Here's how the part is built. I have some questions about the finished solid (model axes, mm). A direction names the side the tool comes from. Give positions to 0.01 mm unless a question says otherwise; leave off trailing zeros. Write each loop counter-clockwise with the first axis right and the second up, starting at its lowest first coordinate (ties: lowest second). Pieces come first, ordered by that corner, then holes. Notation, with made-up numbers: (21, -35) -> (62, -35) arc R14 ccw to (62, -8) -> close; hole circle Ø6 at (-37, 38.5). An arc over 180 degrees is marked (long way). Use one line per item in the form item = value.
```python
from build123d import *

# Parameters (mm, degrees)
BOSS_EXTRUDE1_DEPTH = 56.75
SKETCH2_W           = 5
SKETCH2_H           = 85
SKETCH2_R           = 1.5
CUT_EXTRUDE1_DEPTH  = 2
SKETCH3_R           = 5
CUT_EXTRUDE2_DEPTH  = 3
CHAMFER1_SIZE       = 0.5
CUT_EXTRUDE3_DEPTH  = 5.5
CUT_EXTRUDE4_DEPTH  = 10


with BuildPart() as part:
    # Sketch1 → Boss-Extrude1 (new body, symmetric)
    with BuildSketch(Plane.XY):
        Polygon((0, 50), (0, -50), (7.5, -50), (7.5, -42.5), (2, -42.5), (2, 42.5), (7.5, 42.5), (7.5, 50), align=None)
    extrude(amount=BOSS_EXTRUDE1_DEPTH, both=True)

    # Sketch2 → Cut-Extrude1 (cut)
    with BuildSketch(Plane(origin=(2, 0, 0), x_dir=(0, 0, -1), z_dir=(1, 0, 0))):
        with Locations((-54.25, 0)):
            Rectangle(SKETCH2_W, SKETCH2_H)
        with Locations((54.25, 0)):
            Rectangle(SKETCH2_W, SKETCH2_H)
        with Locations((-47.75, 17.5)):
            Circle(SKETCH2_R)
        with Locations((-47.75, -17.5)):
            Circle(SKETCH2_R)
        with Locations((47.75, 17.5)):
            Circle(SKETCH2_R)
        with Locations((47.75, -17.5)):
            Circle(SKETCH2_R)
    extrude(amount=-CUT_EXTRUDE1_DEPTH, mode=Mode.SUBTRACT)

    # Sketch3 → Cut-Extrude2 (cut, through all)
    with BuildSketch(Plane(origin=(2, 0, 0), x_dir=(0, 0, -1), z_dir=(1, 0, 0))):
        Circle(SKETCH3_R)
        with BuildLine():
            Line((-30.354626116, -39.5), (25.154965406, -39.5))
            ThreePointArc((25.154965406, -39.5), (29.821654194, -36.294997423), (28.505643146, -30.7888063))
            Line((28.505643146, -30.7888063), (7.843483172, -12.13382758))
            ThreePointArc((7.843483172, -12.13382758), (6.353277021, -11.405989443), (4.704093974, -11.58108371))
            ThreePointArc((4.704093974, -11.58108371), (0, -12.5), (-4.704093974, -11.58108371))
            ThreePointArc((-4.704093974, -11.58108371), (-6.353277021, -11.405989443), (-7.843483172, -12.13382758))
            Line((-7.843483172, -12.13382758), (-32.36503276, -34.27328378))
            ThreePointArc((-32.36503276, -34.27328378), (-33.154639389, -37.576998454), (-30.354626116, -39.5))
        make_face()
        with BuildLine():
            Line((-43.75, -27.697319579), (-43.75, 27.697319579))
            ThreePointArc((-43.75, 27.697319579), (-41.968355463, 30.438780862), (-38.739593356, 29.924035799))
            Line((-38.739593356, 29.924035799), (-12.869499782, 6.56703703))
            ThreePointArc((-12.869499782, 6.56703703), (-11.993687913, 5.158698897), (-11.999924538, 3.500258718))
            ThreePointArc((-11.999924538, 3.500258718), (-12.5, 0), (-11.999924538, -3.500258718))
            ThreePointArc((-11.999924538, -3.500258718), (-11.993687913, -5.158698897), (-12.869499782, -6.56703703))
            Line((-12.869499782, -6.56703703), (-38.739593356, -29.924035799))
            ThreePointArc((-38.739593356, -29.924035799), (-41.968355463, -30.438780862), (-43.75, -27.697319579))
        make_face()
        with BuildLine():
            Line((-30.354626116, 39.5), (25.154965406, 39.5))
            ThreePointArc((25.154965406, 39.5), (29.821654194, 36.294997423), (28.505643146, 30.7888063))
            Line((28.505643146, 30.7888063), (7.843483172, 12.13382758))
            ThreePointArc((7.843483172, 12.13382758), (6.353277021, 11.405989443), (4.704093974, 11.58108371))
            ThreePointArc((4.704093974, 11.58108371), (0, 12.5), (-4.704093974, 11.58108371))
            ThreePointArc((-4.704093974, 11.58108371), (-6.353277021, 11.405989443), (-7.843483172, 12.13382758))
            Line((-7.843483172, 12.13382758), (-32.36503276, 34.27328378))
            ThreePointArc((-32.36503276, 34.27328378), (-33.154639389, 37.576998454), (-30.354626116, 39.5))
        make_face()
        with BuildLine():
            Line((43.75, -27.697319579), (43.75, 27.697319579))
            ThreePointArc((43.75, 27.697319579), (41.968355463, 30.438780862), (38.739593356, 29.924035799))
            Line((38.739593356, 29.924035799), (12.869499782, 6.56703703))
            ThreePointArc((12.869499782, 6.56703703), (11.993687913, 5.158698897), (11.999924538, 3.500258718))
            ThreePointArc((11.999924538, 3.500258718), (12.5, 0), (11.999924538, -3.500258718))
            ThreePointArc((11.999924538, -3.500258718), (11.993687913, -5.158698897), (12.869499782, -6.56703703))
            Line((12.869499782, -6.56703703), (38.739593356, -29.924035799))
            ThreePointArc((38.739593356, -29.924035799), (41.968355463, -30.438780862), (43.75, -27.697319579))
        make_face()
        with BuildLine():
            Line((35.25, -39.45), (38.25, -39.45))
            ThreePointArc((38.25, -39.45), (39.8, -41), (38.25, -42.55))
            Line((38.25, -42.55), (35.25, -42.55))
            ThreePointArc((35.25, -42.55), (33.7, -41), (35.25, -39.45))
        make_face()
        with BuildLine():
            Line((35.25, 42.55), (38.25, 42.55))
            ThreePointArc((38.25, 42.55), (39.8, 41), (38.25, 39.45))
            Line((38.25, 39.45), (35.25, 39.45))
            ThreePointArc((35.25, 39.45), (33.7, 41), (35.25, 42.55))
        make_face()
    extrude(amount=-CUT_EXTRUDE2_DEPTH, mode=Mode.SUBTRACT)

    # Chamfer1
    chamfer1_edges = [part.edges().sort_by_distance(p)[0] for p in [
        (0, -50, 0),
        (0, 50, 0),
    ]]
    chamfer(chamfer1_edges, length=CHAMFER1_SIZE)

    # Sketch4 → Cut-Extrude3 (cut)
    with BuildSketch(Plane(origin=(7.5, 0, 0), x_dir=(0, 0, -1), z_dir=(1, 0, 0))):
        with BuildLine():
            Line((42.75, -48), (-42.75, -48))
            ThreePointArc((-42.75, -48), (-45.578427125, -46.828427125), (-46.75, -44))
            Line((-46.75, -44), (-46.75, -43.5))
            ThreePointArc((-46.75, -43.5), (-47.042893219, -42.792893219), (-47.75, -42.5))
            Line((-47.75, -42.5), (47.75, -42.5))
            ThreePointArc((47.75, -42.5), (47.042893219, -42.792893219), (46.75, -43.5))
            Line((46.75, -43.5), (46.75, -44))
            ThreePointArc((46.75, -44), (45.578427125, -46.828427125), (42.75, -48))
        make_face()
        with BuildLine():
            Line((-46.75, 44), (-46.75, 43.5))
            ThreePointArc((-46.75, 43.5), (-47.042893219, 42.792893219), (-47.75, 42.5))
            Line((-47.75, 42.5), (47.75, 42.5))
            ThreePointArc((47.75, 42.5), (47.042893219, 42.792893219), (46.75, 43.5))
            Line((46.75, 43.5), (46.75, 44))
            ThreePointArc((46.75, 44), (45.578427125, 46.828427125), (42.75, 48))
            Line((42.75, 48), (-42.75, 48))
            ThreePointArc((-42.75, 48), (-45.578427125, 46.828427125), (-46.75, 44))
        make_face()
    extrude(amount=-CUT_EXTRUDE3_DEPTH, mode=Mode.SUBTRACT)

    # Sketch5 → Cut-Extrude4 (cut)
    with BuildSketch(Plane.ZY):
        with BuildLine():
            ThreePointArc((-51.75, 27.820508076), (-51.409258263, 30.408698527), (-50.410254038, 32.820508076))
            Line((-50.410254038, 32.820508076), (-48.285898385, 36.5))
            ThreePointArc((-48.285898385, 36.5), (-48.285898385, 40.5), (-51.75, 42.5))
            Line((-51.75, 42.5), (-51.75, 27.820508076))
        make_face()
        with BuildLine():
            ThreePointArc((-50.410254038, -32.820508076), (-51.409258263, -30.408698527), (-51.75, -27.820508076))
            Line((-51.75, -27.820508076), (-51.75, -42.5))
            ThreePointArc((-51.75, -42.5), (-48.285898385, -40.5), (-48.285898385, -36.5))
            Line((-48.285898385, -36.5), (-50.410254038, -32.820508076))
        make_face()
    cut_extrude4 = extrude(amount=-CUT_EXTRUDE4_DEPTH, mode=Mode.SUBTRACT)

    # Mirror1: Cut-Extrude4 across plane
    add(cut_extrude4.mirror(Plane.XY), mode=Mode.SUBTRACT)


solid = part.part
```
Q1. I want a section at C-C, the plane z = 28. Write out the boundary of the cut face in (x, y).
Result set:
outline = (0, -49.5) -> (0.5, -50) -> (7.5, -50) -> (7.5, -48) -> (2, -48) -> (2, -39.5) -> (0, -39.5) -> close; (0, -30.33) -> (2, -30.33) -> (2, -20.23) -> (0, -20.23) -> close; (0, 20.23) -> (2, 20.23) -> (2, 30.33) -> (0, 30.33) -> close; (0, 39.5) -> (2, 39.5) -> (2, 48) -> (7.5, 48) -> (7.5, 50) -> (0.5, 50) -> (0, 49.5) -> close
Q2. I want a section at A-A, the plane x = 3.75. Write out the boundary of the cut face in (y, z).
Result set:
outline = (-50, -56.75) -> (-42.5, -56.75) -> (-42.5, -47.75) arc R1 ccw to (-43.5, -46.75) -> (-44, -46.75) arc R4 cw to (-48, -42.75) -> (-48, 42.75) arc R4 cw to (-44, 46.75) -> (-43.5, 46.75) arc R1 ccw to (-42.5, 47.75) -> (-42.5, 56.75) -> (-50, 56.75) -> close; (42.5, -56.75) -> (50, -56.75) -> (50, 56.75) -> (42.5, 56.75) -> (42.5, 47.75) arc R1 ccw to (43.5, 46.75) -> (44, 46.75) arc R4 cw to (48, 42.75) -> (48, -42.75) arc R4 cw to (44, -46.75) -> (43.5, -46.75) arc R1 ccw to (42.5, -47.75) -> close
Q3. I want a section at B-B, the plane y = -25.5. Write out the boundary of the cut face in (x, z).
Result set:
outline = (0, -51.75) -> (2, -51.75) -> (2, -43.75) -> (0, -43.75) -> close; (0, -33.84) -> (2, -33.84) -> (2, -22.65) -> (0, -22.65) -> close; (0, 22.65) -> (2, 22.65) -> (2, 33.84) -> (0, 33.84) -> close; (0, 43.75) -> (2, 43.75) -> (2, 51.75) -> (0, 51.75) -> close
Q4. Will these pins go through, and if not, where does the flat tip stop? pin 1 Ø0.6 at (x, y) = (1, -4.5) entering from -Z; pin 2 Ø3 at (y, z) = (-40, -2) entering from +X; pin 3 Ø2 at (x, y) = (0.5, 8.5) entering from +Z; pin 4 Ø8 at (y, z) = (0, 0) entering from +X.
Result set:
pin_1 = -51.75
pin_2 = 2
pin_3 = 51.75
pin_4 = through
Q5. If I drill on line 1 along Y through (x, z) = (4, 50); line 2 along Y through (x, z) = (7, -17.5); line 3 along X through (y, z) = (-42, 26), over which ranges is the centre line in solid material (lowest first)? Write a range as from..to.
Result set:
line_1 = -50..-42.5, 42.5..50
line_2 = -50..-48, 48..50
line_3 = 0..2
Q6. Which directions (+Z, -Z, +X, -X, +Y, -Y) give clear straight access to the entire face, cutting with the end or side of a thin tool? Please do faces 1 (the face through (1.01, -21.59, -18.32)), 2 (the face through (0.986, 40.449, -48.257)), 3 (the face through (4.788, 46.859, 45.547)), 4 (the face through (4, 42.5, -52)).
Result set:
face_1 = +X, -X
face_2 = -Z, +X, -X
face_3 = +X
face_4 = -Z, +X
Q7. If we mould it in two halves opening along Y, with no side actions, what happens to faces 5 (the face through (7.5, -49, 1)), 6 (the face through (4, -42.5, 52))? For each: +Y half, -Y half, draft (parallel to the pull), parting line (faces both ways), or undercut.
Result set:
face_5 = draft
face_6 = undercut
Q8. I want a section at D-D, the plane y = -10. Write out the boundary of the cut face in (x, z).
Result set:
outline = (0, -51.75) -> (2, -51.75) -> (2, -43.75) -> (0, -43.75) -> close; (0, -16.67) -> (2, -16.67) -> (2, 16.67) -> (0, 16.67) -> close; (0, 43.75) -> (2, 43.75) -> (2, 51.75) -> (0, 51.75) -> close
